Autodesk Fusion 360 part; units mm, degrees
sketch "Sketch1" plane through (0, 0, 0) normal (0, 0, 1) x (1, 0, 0)
  line L0 (-25.4, 66.675) -> (25.4, 66.675)
  line L1 (25.4, -66.675) -> (-25.4, -66.675)
  circle A0 centre (-8.3186, 12.705) radius 1.59
  circle A1 centre (7.9382, 3.175) radius 3.175
  circle A2 centre (3.17, -5.075) radius 1.995
  arc A3 (-21.5734, -9.515) -> (-25.4, -9.515) centre (-23.4867, -12.055) ccw
  arc A4 (-25.4, -15.875) -> (-21.5734, -15.875) centre (-23.4867, -13.335) ccw
  line L2 (-21.5734, -9.515) -> (0, -9.515)
  arc A5 (0, -15.875) -> (0, -9.515) centre (0, -12.695) ccw
  line L3 (0, -15.875) -> (-21.5734, -15.875)
  line L4 (-25.4, -66.675) -> (-25.4, -15.875)
  line L5 (-25.4, -9.515) -> (-25.4, 66.675)
  arc A6 (25.4, 15.885) -> (21.5734, 15.885) centre (23.4867, 13.345) ccw
  arc A7 (21.5734, 9.525) -> (25.4, 9.525) centre (23.4867, 12.065) ccw
  line L6 (21.5734, 9.525) -> (0, 9.525)
  arc A8 (0, 15.885) -> (0, 9.525) centre (0, 12.705) ccw
  line L7 (0, 15.885) -> (21.5734, 15.885)
  line L8 (25.4, 66.675) -> (25.4, 15.885)
  line L9 (25.4, 9.525) -> (25.4, -66.675)
  line L10 (0, 66.675) -> (0, -66.675) construction
  line L11 (-60, 0) -> (90, 0) construction
  circle A9 centre (0, 41.275) radius 9.145
  circle A10 centre (0, -41.275) radius 9.145
  line L12 (-8.3186, 12.705) -> (0, 12.705) construction
  line L13 (-23.4867, -12.055) -> (-23.4867, -13.335) construction
  line L14 (0, -12.695) -> (-23.4867, -12.695) construction
  line L15 (23.4867, 13.345) -> (23.4867, 12.065) construction
  line L16 (0, 12.705) -> (23.4867, 12.705) construction
  line L17 (-25.4, -9.515) -> (-21.5734, -9.515) construction
  line L18 (21.5734, 15.885) -> (25.4, 15.885) construction
  dimension "d1" = 133.35
  dimension "d2" = 50.8
  dimension "d3" = 3.18
  dimension "d4" = 6.35
  dimension "d5" = 3.99
  dimension "d6" = 3.18
  dimension "d7" = 18.29
  dimension "d8" = 25.4
  dimension "d9" = 25.4
  dimension "d10" = 3.18
  dimension "d11" = 3.18
  dimension "d12" = 53.98
  dimension "d13" = 79.38
  dimension "d14" = 61.6
  dimension "d15" = 69.85
  dimension "d16" = 17.4618
  dimension "d17" = 22.23
  dimension "d18" = 33.7186
  dimension "d19" = 0.64
  dimension "d20" = 0.64
  dimension "d21" = 66.675
extrude "Extrude1" add sketch "Sketch1" along normal mid plane 3.124
Can you work these out from the model? Positions are in its coordinate system, mm. A direction names the side the tool comes from. Round coordinates to 2 decimals unless told otherwise and drop trailing zeros. Loops run counter-clockwise (first coordinate to the right, second up) from the corner with the lowest first, then second, coordinate; pieces in that order, holes last. Notation, with made-up numbers: M -17.75,-8 L 9.25,-8 A16 cw 9.25,-4 Z; hole C 60,6 d6. An arc over 180 degrees is marked long. Write item = value, one per line. Start each with the question number.
(1) Suppose I cut it at C-C on z = 0.8. Write out the boundary of the cut face in (x, y) (3 decimals), plus the area to 3 significant figures.
(2) Suppose I cut it at B-B on y = 37. Write out the boundary of the cut face in (x, z).
(3) Which directions (+Z, -Z, +X, -X, +Y, -Y) give clear straight access to the entire face, cutting with the end or side of a thin tool? Please do faces 4 (the face through (-11, -9.515, 0)), 5 (the face through (11, 15.885, 0)), 6 (the face through (23.458, 16.525, -0.022)).
(4) If we mould it in two halves opening along X, with no side actions, what happens to faces 1 (the face through (-25.4, 28, 0)), 2 (the face through (-3.18, 12.64, -0.02)), 3 (the face through (5.42, 5.11, -0.02))? For each: released by +X, released by -X, zero draft, split by the parting line, or undercut.
(5) Suppose I cut it at A-A on x = -13. Write out the boundary of the cut face in (y, z) (3 decimals), plus the area to 3 significant figures.
(6) I need wall thicknesses on line 1 along Y through (x, z) = (0, 0.05) (3 decimals); line 2 along Y through (x, z) = (-5.5, 1.4) (3 decimals); line 3 along Y through (x, z) = (-20, -0.1) (3 decimals). Which ranges of each line are inside material? Lowest first, please.
Answer block:
q1.outline = M -25.4,-66.675 L 25.4,-66.675 L 25.4,9.525 A3.18 cw 21.573,9.525 L 0,9.525 A3.18 cw 0,15.885 L 21.573,15.885 A3.18 cw 25.4,15.885 L 25.4,66.675 L -25.4,66.675 L -25.4,-9.515 A3.18 cw -21.573,-9.515 L 0,-9.515 A3.18 cw 0,-15.875 L -21.573,-15.875 A3.18 cw -25.4,-15.875 Z; hole C -8.319,12.705 d3.18; hole C 0,-41.275 d18.29; hole C 0,41.275 d18.29; hole C 3.17,-5.075 d3.99; hole C 7.938,3.175 d6.35
q1.area = 5,840 mm²
q2.outline = M -25.4,-1.56 L -8.08,-1.56 L -8.08,1.56 L -25.4,1.56 Z; M 8.08,-1.56 L 25.4,-1.56 L 25.4,1.56 L 8.08,1.56 Z
q3.face_4 = +Z, -Z, -X
q3.face_5 = +Z, -Z, +X
q3.face_6 = +Z, -Z
q4.face_1 = released by -X
q4.face_2 = released by +X
q4.face_3 = undercut
q5.outline = M -66.675,-1.562 L -15.875,-1.562 L -15.875,1.562 L -66.675,1.562 Z; M -9.515,-1.562 L 66.675,-1.562 L 66.675,1.562 L -9.515,1.562 Z
q5.area = 397 mm²
q6.line_1 = -66.675 to -50.42, -32.13 to -15.875, -9.515 to 9.525, 15.885 to 32.13, 50.42 to 66.675
q6.line_2 = -66.675 to -48.581, -33.969 to -15.875, -9.515 to 33.969, 48.581 to 66.675
q6.line_3 = -66.675 to -15.875, -9.515 to 66.675
